Here's how the part is built. I have some questions about the finished solid (model axes, mm). Face numbers are marked on the shaded views. Coordinates: 2 decimals unless noted, no trailing zeros. Write each loop counter-clockwise with the first axis right and the second up, starting at its lowest first coordinate (ties: lowest second). Pieces come first, ordered by that corner, then holes.
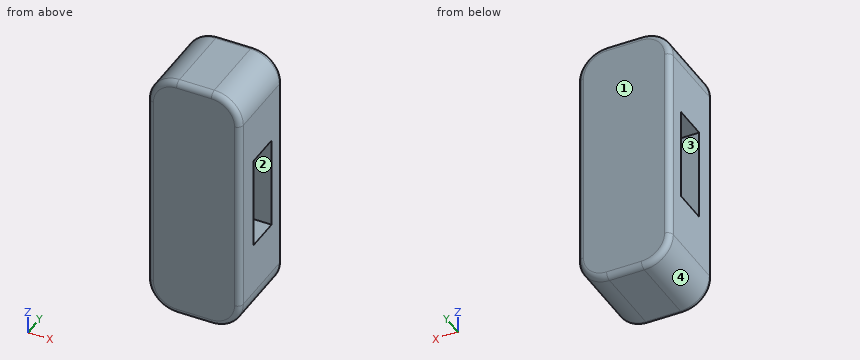
```python
from build123d import *

# Parameters (mm, degrees)
F1_DEPTH = 44.45
F2_R     = 3.175
F3_W     = 19.05
F3_H     = 50.8
F4_DEPTH = 127


with BuildPart() as f1:
    # F0 (on Front) → F1 (new body)
    with BuildSketch(Plane.XZ):
        with BuildLine():
            Line((9.525, 69.85), (-9.525, 69.85))
            ThreePointArc((-9.525, 69.85), (-20.75032, 65.20032), (-25.4, 53.975))
            Line((-25.4, 53.975), (-25.4, -53.975))
            ThreePointArc((-25.4, -53.975), (-20.75032, -65.20032), (-9.525, -69.85))
            Line((-9.525, -69.85), (9.525, -69.85))
            ThreePointArc((9.525, -69.85), (20.75032, -65.20032), (25.4, -53.975))
            Line((25.4, -53.975), (25.4, 53.975))
            ThreePointArc((25.4, 53.975), (20.75032, 65.20032), (9.525, 69.85))
        make_face()
    extrude(amount=F1_DEPTH)

    # F2
    f2_edges = [f1.edges().sort_by_distance(p)[0] for p in [
        (-25.4, -44.45, 0),
        (25.4, 0, 0),
    ]]
    fillet(f2_edges, radius=F2_R)

    # F3 (on Right) → F4 (cut, symmetric)
    with BuildSketch(Plane.YZ):
        with Locations((-20.957332, 0)):
            Rectangle(F3_W, F3_H)
    extrude(amount=F4_DEPTH, both=True, mode=Mode.SUBTRACT)


solid = f1.part
```
1) Imagine slicing it at B-B on z = -3.5. Please give me the cut outline in (x, y) (3 decimals), then the cut area to 3 significant figures.
Values follow:
outline: (-25.4, -41.275) arc R3.175 ccw to (-22.225, -44.45) - (22.225, -44.45) arc R3.175 ccw to (25.4, -41.275) - (25.4, -30.482) - (-25.4, -30.482) - close; (-25.4, -11.432) - (25.4, -11.432) - (25.4, -3.175) arc R3.175 ccw to (22.225, 0) - (-22.225, 0) arc R3.175 ccw to (-25.4, -3.175) - close
area: 1,280 mm2
2) We'd pull the mould along Z, two halves only. Please class the marked faces 1, 2, 3 and 4: pulls with the +Z half, pulls with the -Z half, needs draft (parallel to the pull), parting line crosses it, or undercut.
Values follow:
face 1: needs draft
face 2: undercut
face 3: undercut
face 4: pulls with the -Z half
3) I need wall thicknesses on probe 1 along Z at (x, y) = (5, -15); probe 2 along Y at (x, z) = (7, 17.5); probe 3 along Z at (x, y) = (22, -13.5). Which ranges of each line are inside material? Lowest first, please.
Values follow:
probe 1: z = -69.85 to -25.4, 25.4 to 69.85
probe 2: y = -44.45 to -30.48, -11.43 to 0
probe 3: z = -63.79 to -25.4, 25.4 to 63.79
4) Imagine slicing it at A-A on y = -24. Please give me the cut outline in (x, z) (3 decimals), then the cut area to 3 significant figures.
Values follow:
outline: (-25.4, -53.975) arc R15.875 ccw to (-9.525, -69.85) - (9.525, -69.85) arc R15.875 ccw to (25.4, -53.975) - (25.4, -25.4) - (-25.4, -25.4) - close; (-25.4, 25.4) - (25.4, 25.4) - (25.4, 53.975) arc R15.875 ccw to (9.525, 69.85) - (-9.525, 69.85) arc R15.875 ccw to (-25.4, 53.975) - close
area: 4,300 mm2
5) Imagine slicing it at C-C on x = 2. Please give me the cut outline in (y, z) (3 decimals), then the cut area to 3 significant figures.
Values follow:
outline: (-44.45, -66.675) arc R3.175 ccw to (-41.275, -69.85) - (-3.175, -69.85) arc R3.175 ccw to (0, -66.675) - (0, 66.675) arc R3.175 ccw to (-3.175, 69.85) - (-41.275, 69.85) arc R3.175 ccw to (-44.45, 66.675) - close; hole (-30.482, -25.4) - (-11.432, -25.4) - (-11.432, 25.4) - (-30.482, 25.4) - close
area: 5,230 mm2
6) Will these pins go through, and if not, where does the flat tip stop? pin 1 (1.5 mm diameter, centred on x = 12, y = -9.5, fed in from -Z); pin 2 (12 mm diameter, centred on x = 18, y = -7, fed in from +Z); pin 3 (15 mm diameter, centred on x = -11, y = -25.5, fed in from +Z).
Values follow:
pin 1: stops at z = -69.76
pin 2: stops at z = 69.66
pin 3: stops at z = 69.85
